Check sheet for the modelled part. Datum: model origin and axes. Units: mm. Round coordinates to 2 decimals unless told otherwise and drop trailing zeros. Order: outer loops, then holes, each group sorted by start corner. A loop starts at its lowest first (then second) coordinate and runs counter-clockwise, first axis right, second up. Notation, with made-up numbers: M -26.75,-28 L 6.25,-28 A26 cw 6.25,-10 Z; hole C 32.25,32.25 d2. An arc over 180 degrees is marked long. One line per item, written item: value. Start each with the question number.
(1) Cross-section at B-B, the plane x = -8.5. Enter the section's corners in (y, z).
(2) Depth check by flat-ended pin: pin 1 Ø0.9 at (x, z) = (80.5, 1.5) entering from -Y; pin 2 Ø0.9 at (y, z) = (-6, 1.5) entering from -X; pin 3 Ø3 at (x, y) = (48.11, -7.95) entering from -Z. Enter the tip coordinate at first touch or a pass-through.
(3) Cross-section at A-A, the plane z = 2.5. Count the separate pieces of the cut face and the enclosed holes in it, and give its area (3 significant figures).
(4) Thickness scan on L1, parallel to X at y = -3.5, z = 1.55; L2, parallel to Y at x = -50.5, z = 0.4; L3, parallel to Y at x = -30, z = 2.7. Record the ranges inside material, lowest first.
from build123d import *

# Parameters (mm, degrees)
F0_W     = 253.9
F0_H     = 6.4
F1_DEPTH = 3
F3_DEPTH = 3
F4_R     = 2.63999


# Not quite as in the source:
# - a fillet or chamfer is up to 0.001 mm smaller than in the source, because OpenCascade refuses the exact size


with BuildPart() as f1:
    # F0 (on Top) → F1 (new body)
    with BuildSketch(Plane.XY):
        Rectangle(F0_W, F0_H)
    extrude(amount=F1_DEPTH)

    # F2 (on Top) → F3 (join)
    with BuildSketch(Plane.XY):
        with BuildLine():
            Line((126.95, -10.59), (126.95, -3.2))
            Line((126.95, -3.2), (121.67, -3.2))
            Line((121.67, -3.2), (121.67, -7.95))
            Line((121.67, -7.95), (122.46, -7.95))
            ThreePointArc((122.46, -7.95), (124.31, -6.1), (126.16, -7.95))
            ThreePointArc((126.16, -7.95), (125.6181475452, -9.2581475452), (124.31, -9.8))
            Line((124.31, -9.8), (124.31, -10.59))
            Line((124.31, -10.59), (126.95, -10.59))
        make_face()
        with BuildLine():
            Line((122.46, -7.95), (121.67, -7.95))
            Line((121.67, -7.95), (121.67, -10.59))
            Line((121.67, -10.59), (124.31, -10.59))
            Line((124.31, -10.59), (124.31, -9.8))
            ThreePointArc((124.31, -9.8), (123.0018524548, -9.2581475452), (122.46, -7.95))
        make_face()
        Polygon((50.75, -10.59), (50.75, -3.2), (45.47, -3.2), (45.47, -7.95), (45.47, -10.59), align=None)
        with BuildLine():
            ThreePointArc((49.96, -7.95), (48.11, -9.8), (46.26, -7.95))
            ThreePointArc((46.26, -7.95), (48.11, -6.1), (49.96, -7.95))
        make_face(mode=Mode.SUBTRACT)
        Polygon((-101.65, -3.2), (-106.93, -3.2), (-106.93, -7.95), (-106.93, -10.59), (-101.65, -10.59), align=None)
        with BuildLine():
            ThreePointArc((-102.44, -7.95), (-104.29, -9.8), (-106.14, -7.95))
            ThreePointArc((-106.14, -7.95), (-104.29, -6.1), (-102.44, -7.95))
        make_face(mode=Mode.SUBTRACT)
        Polygon((-25.45, -3.2), (-30.73, -3.2), (-30.73, -7.95), (-30.73, -10.59), (-25.45, -10.59), align=None)
        with BuildLine():
            ThreePointArc((-26.24, -7.95), (-28.09, -9.8), (-29.94, -7.95))
            ThreePointArc((-29.94, -7.95), (-28.09, -6.1), (-26.24, -7.95))
        make_face(mode=Mode.SUBTRACT)
    extrude(amount=F3_DEPTH)

    # F4 (radius 2.64 in the source; OpenCascade refuses exactly that, so slightly less here)
    f4_edges = [f1.edges().sort_by_distance(p)[0] for p in [
        (45.47, -10.59, 1.5),
        (50.75, -10.59, 1.5),
        (121.67, -10.59, 1.5),
        (126.95, -10.59, 1.5),
        (-30.73, -10.59, 1.5),
        (-25.45, -10.59, 1.5),
        (-106.93, -10.59, 1.5),
        (-101.65, -10.59, 1.5),
    ]]
    fillet(f4_edges, radius=F4_R)


solid = f1.part
Values found:
1. outline: M -3.2,0 L 3.2,0 L 3.2,3 L -3.2,3 Z
2. pin 1: y = -3.2
2. pin 2: x = -106.93
2. pin 3: through
3. separate pieces: 1
3. enclosed holes: 4
3. area: 1,730 mm^2
4. L1: -106.93 to -101.65, -30.73 to -25.45, 45.47 to 50.75, 121.67 to 126.95
4. L2: -3.2 to 3.2
4. L3: -9.77 to 3.2
